```python
from build123d import *

# Parameters (mm, degrees)
SKETCH1_R            = 39
SKETCH1_R_2          = 26.5
BOSS_EXTRUDE1_DEPTH  = 1.5
SKETCH3_W            = 50
SKETCH3_H            = 51.5
BOSS_EXTRUDE2_DEPTH  = 1.5
BOSS_EXTRUDE4_DEPTH  = 1.5
SKETCH2_R            = 2.75
CUT_EXTRUDE1_DEPTH   = 2.5
CIRPATTERN1_COUNT    = 6
CUT_EXTRUDE2_START   = -4
SKETCH5_R            = 2.25
CUT_EXTRUDE2_DEPTH   = 5
LPATTERN1_COUNT      = 2
LPATTERN1_PITCH      = 15
LPATTERN1_COUNT_DIR2 = 2
LPATTERN1_PITCH_DIR2 = 10
LPATTERN2_COUNT      = 2
LPATTERN2_PITCH      = 15
LPATTERN2_COUNT_DIR2 = 2
LPATTERN2_PITCH_DIR2 = 10
CUT_EXTRUDE3_START   = -4
SKETCH7_R            = 4.25
CUT_EXTRUDE3_DEPTH   = 5
LPATTERN3_COUNT      = 3
LPATTERN3_PITCH      = 20


with BuildPart() as part:
    # Sketch1 → Boss-Extrude1 (new body, symmetric)
    with BuildSketch(Plane(origin=(0, 0, 0), x_dir=(1, 0, 0), z_dir=(0, 1, 0))):
        Circle(SKETCH1_R)
        Circle(SKETCH1_R_2, mode=Mode.SUBTRACT)
    extrude(amount=BOSS_EXTRUDE1_DEPTH, both=True)

    # Sketch3 → Boss-Extrude2 (add, symmetric)
    with BuildSketch(Plane(origin=(0, 0, 0), x_dir=(1, 0, 0), z_dir=(0, 1, 0))):
        with Locations((0, 52.25)):
            Rectangle(SKETCH3_W, SKETCH3_H)
    extrude(amount=BOSS_EXTRUDE2_DEPTH, both=True)

    # Sketch6 → Boss-Extrude4 (add, symmetric)
    with BuildSketch(Plane(origin=(0, 0, 0), x_dir=(1, 0, 0), z_dir=(0, 1, 0))):
        Polygon((-45, 166.5), (-45, 26.5), (-39, 0), (-14.981514186, 26.5), (16.520833333, 26.5), (39, 0), (45, 26.5), (45, 166.5), align=None)
    extrude(amount=BOSS_EXTRUDE4_DEPTH, both=True)

    # Sketch2 → Cut-Extrude1 (cut, symmetric)
    with BuildSketch(Plane(origin=(0, 0, 0), x_dir=(1, 0, 0), z_dir=(0, 1, 0))):
        with Locations((0, 32.5)):
            Circle(SKETCH2_R)
    cut_extrude1 = extrude(amount=CUT_EXTRUDE1_DEPTH, both=True, mode=Mode.SUBTRACT)

    # CirPattern1: Cut-Extrude1 ×6 about axis
    cirpattern1_axis = Axis((0, 0, 0), (0, 1, 0))
    for i in range(1, CIRPATTERN1_COUNT):
        add(cut_extrude1.rotate(cirpattern1_axis, i * 360 / CIRPATTERN1_COUNT), mode=Mode.SUBTRACT)

    # Sketch5 → Cut-Extrude2 (cut)
    with BuildSketch(Plane(origin=(0, 1.5, 0), x_dir=(1, 0, 0), z_dir=(0, 1, 0)).offset(CUT_EXTRUDE2_START)):
        with Locations((0, 73)):
            Circle(SKETCH5_R)
    cut_extrude2 = extrude(amount=CUT_EXTRUDE2_DEPTH, mode=Mode.SUBTRACT)

    # LPattern1: Cut-Extrude2 2 × 2
    with Locations(*[(i * LPATTERN1_PITCH, 0, j * LPATTERN1_PITCH_DIR2) for i in range(LPATTERN1_COUNT) for j in range(LPATTERN1_COUNT_DIR2) if (i, j) != (0, 0)]):
        add(cut_extrude2, mode=Mode.SUBTRACT)

    # LPattern2: Cut-Extrude2 2 × 2
    with Locations(*[(-i * LPATTERN2_PITCH, 0, j * LPATTERN2_PITCH_DIR2) for i in range(LPATTERN2_COUNT) for j in range(LPATTERN2_COUNT_DIR2) if (i, j) != (0, 0)]):
        add(cut_extrude2, mode=Mode.SUBTRACT)

    # Sketch7 → Cut-Extrude3 (cut)
    with BuildSketch(Plane(origin=(0, 1.5, 0), x_dir=(1, 0, 0), z_dir=(0, 1, 0)).offset(CUT_EXTRUDE3_START)):
        with Locations((-20, 146.5)):
            Circle(SKETCH7_R)
        with Locations((20, 146.5)):
            Circle(SKETCH7_R)
    cut_extrude3 = extrude(amount=CUT_EXTRUDE3_DEPTH, mode=Mode.SUBTRACT)

    # LPattern3: Cut-Extrude3 ×3
    with Locations(*[(0, 0, i * LPATTERN3_PITCH) for i in range(1, LPATTERN3_COUNT)]):
        add(cut_extrude3, mode=Mode.SUBTRACT)


solid = part.part
```
Input: part model. Units: mm. Frame: model coordinates. Round coordinates to 2 decimals unless told otherwise and drop trailing zeros. Loops run counter-clockwise (first coordinate to the right, second up) from the corner with the lowest first, then second, coordinate; pieces in that order, holes last.
1) Section query A-A on z = -32.5. Return the cut outline in (x, y), plus the area to 4 significant figures.
Ans:
outline: (-45, -1.5) - (-2.75, -1.5) - (-2.75, 1.5) - (-45, 1.5) - close; (2.75, -1.5) - (45, -1.5) - (45, 1.5) - (2.75, 1.5) - close
area: 253.5 mm2
2) Material intervals for line 1 (Z direction, x = 0, y = 0.8); line 2 (Z direction, x = -20, y = -0.05); line 3 (Z direction, x = 23.5, y = -0.15), sorted ascending.
Ans:
line 1: z = -166.5 to -75.25, -70.75 to -65.25, -60.75 to -35.25, -29.75 to -26.5, 26.5 to 29.75, 35.25 to 39
line 2: z = -166.5 to -150.75, -142.25 to -130.75, -122.25 to -110.75, -102.25 to -17.39, 17.39 to 33.48
line 3: z = -166.5 to -148.91, -144.09 to -128.91, -124.09 to -108.91, -104.09 to -12.25, 12.25 to 31.12
3) Section query C-C on x = 0. Return the cut outline in (y, z).
Ans:
outline: (-1.5, -166.5) - (1.5, -166.5) - (1.5, -75.25) - (-1.5, -75.25) - close; (-1.5, -70.75) - (1.5, -70.75) - (1.5, -65.25) - (-1.5, -65.25) - close; (-1.5, -60.75) - (1.5, -60.75) - (1.5, -35.25) - (-1.5, -35.25) - close; (-1.5, -29.75) - (1.5, -29.75) - (1.5, -26.5) - (-1.5, -26.5) - close; (-1.5, 26.5) - (1.5, 26.5) - (1.5, 29.75) - (-1.5, 29.75) - close; (-1.5, 35.25) - (1.5, 35.25) - (1.5, 39) - (-1.5, 39) - close
4) Section query D-D on z = -126.5. Return the cut outline in (x, y), plus the area to 3 significant figures.
Ans:
outline: (-45, -1.5) - (-24.25, -1.5) - (-24.25, 1.5) - (-45, 1.5) - close; (-15.75, -1.5) - (15.75, -1.5) - (15.75, 1.5) - (-15.75, 1.5) - close; (24.25, -1.5) - (45, -1.5) - (45, 1.5) - (24.25, 1.5) - close
area: 219 mm2
5) Pin query (flat end, axial travel): pin 1 (5 mm diameter, centred on x = -28.15, z = 16.25, fed in from +Y); pin 2 (1 mm diameter, centred on y = 0.5, z = -17, fed in from -X). Return the tip coordinate at first contact, or that it passes through.
Ans:
pin 1: passes through
pin 2: stops at x = -42.96
6) Pull-direction query (X, two-part tool) for faces 1 (the cylindrical face through (-20.553, -0.021, -110.714)), 2 (the flat face through (41.958, 0.021, -13.065)), 3 (the cylindrical face through (14.246, -0.021, -22.345)), 4 (the flat face through (-1, 1.5, -88)); classes: released by +X, released by -X, zero draft, split by the parting line, or undercut.
Ans:
face 1: undercut
face 2: released by +X
face 3: undercut
face 4: zero draft
7) Section query B-B on z = -63. Return the cut outline in (x, y).
Ans:
outline: (-45, -1.5) - (-17.25, -1.5) - (-17.25, 1.5) - (-45, 1.5) - close; (-12.75, -1.5) - (-2.25, -1.5) - (-2.25, 1.5) - (-12.75, 1.5) - close; (2.25, -1.5) - (12.75, -1.5) - (12.75, 1.5) - (2.25, 1.5) - close; (17.25, -1.5) - (45, -1.5) - (45, 1.5) - (17.25, 1.5) - close
